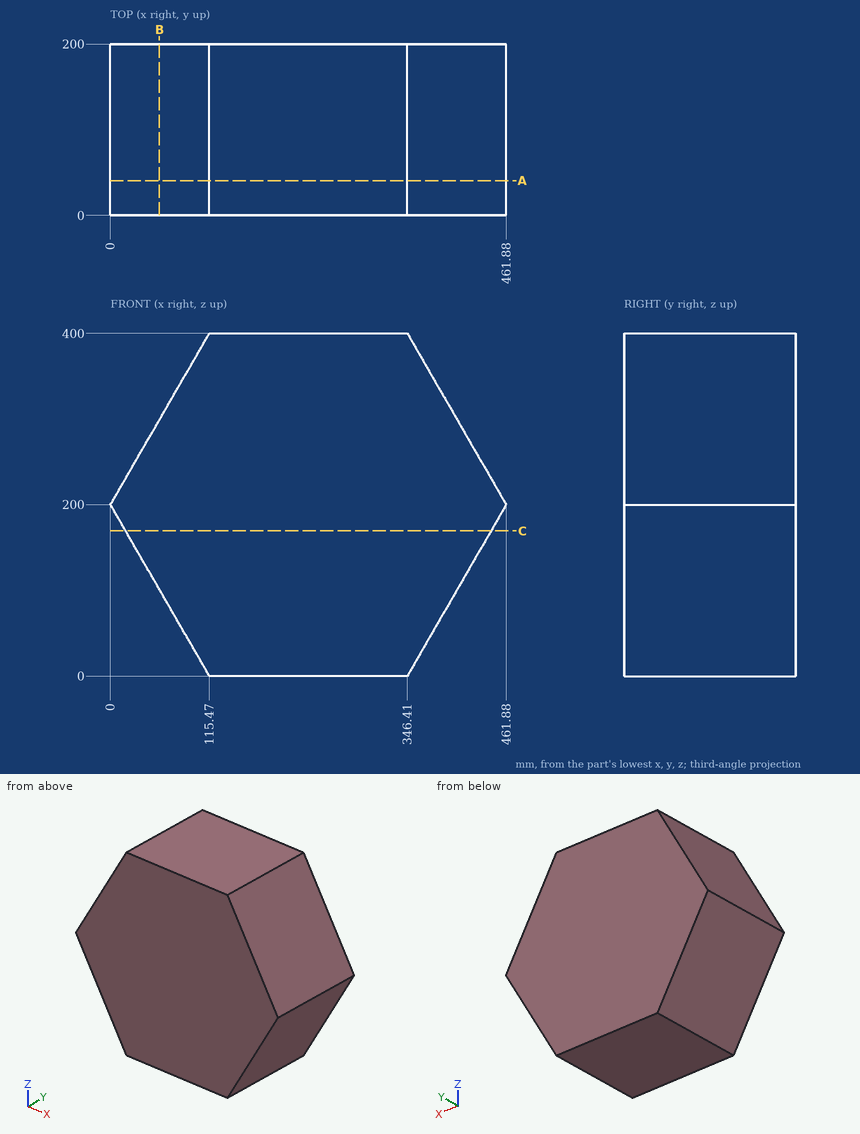
Job drawing, mm, ordinate dimensions from the low corner. One solid piece. Coordinates: 2 decimals unless noted, no trailing zeros. Loops run counter-clockwise (first coordinate to the right, second up) from the corner with the lowest first, then second, coordinate; pieces in that order, holes last. Notation, with made-up numbers: (33, -25) - (47, -25) arc R27 cw to (47, -4) - close; hole circle Ø1 at (9.25, 39.5). An arc over 180 degrees is marked (long way). Answer as a JSON object with one key per item and string values. Group by question number.
(1) Cut at A-A (y = 40.5). Give the cut face in (x, z).
(2) Flat gauge pins, fed straight in: pin 1 (10 mm diameter, centred on y = 26, z = 187, fed in from +X); pin 2 (3 mm diameter, centred on y = 160.5, z = 138, fed in from -X); pin 3 (8 mm diameter, centred on y = 58.5, z = 115, fed in from +X) (1 decimal). Where does each tip first touch, or does it go through?
(3) Cut at B-B (x = 57). Give the cut face in (y, z), then the cut area to 3 significant figures.
(4) Cut at C-C (z = 169.5). Give the cut face in (x, y).
(5) Probe line 1 along Z through (x, y) = (28.5, 33) (1 decimal); line 2 along X through (y, z) = (58, 58.5) (1 decimal); line 3 along Z through (x, y) = (418.5, 47) (1 decimal). List the from-to ranges inside material, lowest first.
Geometry says:
{
 "1": {"outline": "(0, 200) - (115.47, 0) - (346.41, 0) - (461.88, 200) - (346.41, 400) - (115.47, 400) - close"},
 "2": {"pin 1": "stops at x = 457.26", "pin 2": "stops at x = 34.93", "pin 3": "stops at x = 415.1"},
 "3": {"outline": "(0, 101.27) - (200, 101.27) - (200, 298.73) - (0, 298.73) - close", "area": "39,500 mm^2"},
 "4": {"outline": "(17.61, 0) - (444.27, 0) - (444.27, 200) - (17.61, 200) - close"},
 "5": {"line 1": "z = 150.6 to 249.4", "line 2": "x = 81.7 to 380.2", "line 3": "z = 124.9 to 275.1"}
}
